from build123d import *


with BuildPart() as part:
    # Эскиз1 → Повернуть1 (revolve)
    with BuildSketch(Plane.XY):
        with BuildLine():
            Line((5.673835343, 75.737111548), (0, 74.5635))
            Line((0, 74.5635), (0, 88))
            ThreePointArc((0, 88), (0.585786438, 89.414213562), (2, 90))
            Line((2, 90), (41, 90))
            ThreePointArc((41, 90), (42.414213562, 89.414213562), (43, 88))
            Line((43, 88), (43, 83.457888633))
            Line((43, 83.457888633), (38.55204573, 82.537845984))
            Line((38.55204573, 82.537845984), (43, 66.589154016))
            Line((43, 66.589154016), (43, 66.789154016))
            Line((43, 66.789154016), (55.8, 66.789154016))
            ThreePointArc((55.8, 66.789154016), (55.941421356, 66.730575372), (56, 66.589154016))
            Line((56, 66.589154016), (56, 55.2))
            ThreePointArc((56, 55.2), (55.941421356, 55.058578644), (55.8, 55))
            Line((55.8, 55), (0.2, 55))
            ThreePointArc((0.2, 55), (0.058578644, 55.058578644), (0, 55.2))
            Line((0, 55.2), (0, 55.392870878))
            Line((0, 55.392870878), (11.347670687, 55.392870878))
            Line((11.347670687, 55.392870878), (5.673835343, 75.737111548))
        make_face()
    revolve(axis=Axis((-882.527700014, 0, 0), (1, 0, 0)))


solid = part.part
Model file for the job. Use its own axes, mm. A direction names the side the tool comes from. Coordinates: 2 decimals unless noted, no trailing zeros. Order: outer loops, then holes, each group sorted by start corner. A loop starts at its lowest first (then second) coordinate and runs counter-clockwise, first axis right, second up. Notation, with made-up numbers: M 3.5,55 L 13.5,55 A5 ccw 13.5,59 Z; hole C 22,38 d6. An arc over 180 degrees is marked long. Return JSON: item names as keys, results as strings.
1. Saw through at B-B (x = 8). Give the cut face in (y, z), and give its area (3 significant figures).
Ans:
{"outline": "C 0,0 d180; C 0,0 d110.79; hole C 0,0 d134.79; hole C 0,0 d110", "area": "11,300 mm^2"}
2. Saw through at C-C (x = 47). Give the cut face in (y, z).
Ans:
{"outline": "C 0,0 d133.58; hole C 0,0 d110"}
3. Tool access for faces 1 (the face through (5.753, -43.958, -33.706)), 2 (the face through (49.49, 63.705, 20.062)), 3 (the face through (0.275, 34.433, -66.201)): list every direction of +Z, -Z, +X, -X, +Y, -Y with a clear straight run to the whole face (end or side of a thin tool).
Ans:
{"face 1": "-X", "face 2": "+X", "face 3": "none"}
4. Pull direction Z, two halves, no side cores. Call faces 4 (the face through (42.784, -8.769, 66.79)), 5 (the face through (56, -25, 50)), 6 (the face through (21.773, 41.53, -79.845)): +Z half, -Z half, draft (parallel to the pull), parting line (faces both ways), or undercut.
Ans:
{"face 4": "undercut", "face 5": "draft", "face 6": "parting line"}
5. Drill centre lines: probe 1 along Y at (x, z) = (48.5, -1); probe 2 along Z at (x, y) = (38, 0); probe 3 along Z at (x, y) = (44, 0). Where is each one in solid material? Low to high.
Ans:
{"probe 1": "-66.78 to -54.99, 54.99 to 66.78", "probe 2": "-90 to -55, 55 to 90", "probe 3": "-66.79 to -55, 55 to 66.79"}
6. Flat gauge pins, fed straight in: pin 1 (10 mm diameter, centred on x = 11.5, y = -49, fed in from +Z); pin 2 (3 mm diameter, centred on x = 36.5, y = 61.5, fed in from +Z); pin 3 (1.5 mm diameter, centred on y = 65.5, z = 9.5, fed in from -X). Where does each tip first touch, or does it go through?
Ans:
{"pin 1": "z = 78.51", "pin 2": "z = 67.08", "pin 3": "x = 8.13"}
7. Saw through at A-A (x = 36). Give the cut face in (y, z), and give its area (3 significant figures).
Ans:
{"outline": "C 0,0 d180; hole C 0,0 d110", "area": "15,900 mm^2"}
